```python
from build123d import *

# Parameters (mm, degrees)
SKETCH2_W           = 4
SKETCH2_H           = 30
BOSS_EXTRUDE1_DEPTH = 25
SKETCH3_W           = 1
SKETCH3_H           = 38
CUT_EXTRUDE1_DEPTH  = 34


with BuildPart() as part:
    # Sketch2 → Boss-Extrude1 (new body)
    with BuildSketch(Plane(origin=(0, 0, 0), x_dir=(0, 0, -1), z_dir=(1, 0, 0))):
        Rectangle(SKETCH2_W, SKETCH2_H)
        Polygon((-2, 19), (-2, 15), (2, 15), (36, 15), (36, 19), align=None)
        Polygon((2, -15), (-2, -15), (-2, -19), (36, -19), (36, -15), align=None)
    extrude(amount=BOSS_EXTRUDE1_DEPTH)

    # Sketch3 → Cut-Extrude1 (cut)
    with BuildSketch(Plane.XY.offset(2)):
        with Locations((3.469945018, 0)):
            Rectangle(SKETCH3_W, SKETCH3_H)
        with Locations((21.530054982, 0)):
            Rectangle(SKETCH3_W, SKETCH3_H)
    extrude(amount=-CUT_EXTRUDE1_DEPTH, mode=Mode.SUBTRACT)


solid = part.part
```
Here's how the part is built. I have some questions about the finished solid (model axes, mm). A direction names the side the tool comes from. Round coordinates to 2 decimals unless told otherwise and drop trailing zeros. Order: outer loops, then holes, each group sorted by start corner. A loop starts at its lowest first (then second) coordinate and runs counter-clockwise, first axis right, second up. Notation, with made-up numbers: (69.25, 0) -> (126.25, 0) arc R25 cw to (126.25, 20) -> close; hole circle Ø2 at (-29.5, -20.75). An arc over 180 degrees is marked (long way). Use a Markdown table: item, result. Add a question column.
(1) If we mould it in two halves opening along Y, with no side actions, what happens to faces 4 (the face through (12, 19, -17)), 5 (the face through (12, -15, -19)), 6 (the face through (12, -17, -36))? For each: released by +Y, released by -Y, zero draft, split by the parting line, or undercut.
(2) Suppose I cut it at B-B, the plane y = 3.5. Please give me the cut outline in (x, z), and give its area (3 significant figures).
(3) Suppose I cut it at C-C, the plane x = 12.75. Please give me the cut outline in (y, z), and give its area (3 significant figures).
(4) For faces 1 (the face through (0, 0, -1)), 2 (the face through (2.97, -1, -1)), 3 (the face through (23, 0, -2)), which set-ups out of +Z, -Z, +X, -X, +Y, -Y let a thin tool reach every point of the face, with its end or its side?
(5) Suppose I cut it at A-A, the plane z = -33.5. Please give me the cut outline in (x, y), and give its area (3 significant figures).
(6) For pin 1 Ø3.5 at (x, y) = (1.5, -2) entering from -Z; pin 2 Ø0.5 at (x, y) = (3.5, 17.5) entering from +Z, each with a flat end and sliding along its axis, tell me the tip position at first contact or that it passes through.
(7) Suppose I cut it at D-D, the plane z = -5. Please give me the cut outline in (x, y).
(8) I need wall thicknesses on line 1 along X through (y, z) = (7, -1); line 2 along Y through (x, z) = (12.75, -27); line 3 along Z through (x, y) = (11.75, -7). Which ranges of each line are inside material? Lowest first, please.
Verdict:
| question | item | result |
|---|---|---|
| 1 | face 4 | released by +Y |
| 1 | face 5 | undercut |
| 1 | face 6 | zero draft |
| 2 | outline | (0, -2) -> (2.97, -2) -> (2.97, 2) -> (0, 2) -> close; (3.97, -2) -> (21.03, -2) -> (21.03, 2) -> (3.97, 2) -> close; (22.03, -2) -> (25, -2) -> (25, 2) -> (22.03, 2) -> close |
| 2 | area | 92.0 mm2 |
| 3 | outline | (-19, -36) -> (-15, -36) -> (-15, -2) -> (15, -2) -> (15, -36) -> (19, -36) -> (19, 2) -> (-19, 2) -> close |
| 3 | area | 424 mm2 |
| 4 | face 1 | +Z, -Z, -X, +Y, -Y |
| 4 | face 2 | +Z, +Y, -Y |
| 4 | face 3 | -Z, +X, -X |
| 5 | outline | (0, -19) -> (25, -19) -> (25, -15) -> (0, -15) -> close; (0, 15) -> (25, 15) -> (25, 19) -> (0, 19) -> close |
| 5 | area | 200 mm2 |
| 6 | pin 1 | z = -2 |
| 6 | pin 2 | z = -32 |
| 7 | outline | (0, -19) -> (2.97, -19) -> (2.97, -15) -> (0, -15) -> close; (0, 15) -> (2.97, 15) -> (2.97, 19) -> (0, 19) -> close; (3.97, -19) -> (21.03, -19) -> (21.03, -15) -> (3.97, -15) -> close; (3.97, 15) -> (21.03, 15) -> (21.03, 19) -> (3.97, 19) -> close; (22.03, -19) -> (25, -19) -> (25, -15) -> (22.03, -15) -> close; (22.03, 15) -> (25, 15) -> (25, 19) -> (22.03, 19) -> close |
| 8 | line 1 | 0 to 2.97, 3.97 to 21.03, 22.03 to 25 |
| 8 | line 2 | -19 to -15, 15 to 19 |
| 8 | line 3 | -2 to 2 |
